Verification items for the finished model (mm, model axes). A direction names the side the tool comes from. Give positions to 0.01 mm unless a question says otherwise; leave off trailing zeros. Loops run counter-clockwise (first coordinate to the right, second up) from the corner with the lowest first, then second, coordinate; pieces in that order, holes last. Notation, with made-up numbers: (-25.5, 54.25) - (-19.5, 54.25) arc R17 cw to (-19.5, 74.25) - close; hole circle Ø6 at (89, -23.75). An arc over 180 degrees is marked (long way). One line per item, written item: value. Start each with the question number.
1. Scan lines: L1, parallel to Z at x = 0, y = 6.5; L2, parallel to X at y = 8, z = -195; L3, parallel to X at y = 7, z = 0. Record each from-to range of solid material in increasing order. Write a range as [from, to].
2. Access from +Z, -Z, +X, -X, +Y, -Y to the whole of each face (thin tool, end or side, straight path). Record for faces 5 (the flat face through (2, 3, 228)), 6 (the cylindrical face through (229, 2, 169)), 7 (the flat face through (120, 5, 231)).
3. Gauge pin test, flat ends, axial feed: pin 1 (13 mm diameter, centred on x = 0, z = -45, fed in from +Y); pin 2 (12 mm diameter, centred on x = -34, y = -54, fed in from +Z); pin 3 (5 mm diameter, centred on y = 7.5, z = -157, fed in from -X); pin 4 (11 mm diameter, centred on y = 5, z = -149, fed in from +X). Record the tip position at first contact, or that the pin passes through.
4. Sectioned sample at C-C (y = -34). Record the cut outline in (x, z), plus the area to 3 significant figures.
5. Mould release check, pull along X, two halves, no side actions. Record for faces 1 (the flat face through (228, 3, 163)), 2 (the flat face through (-120, 5, 231)), 3 (the cylindrical face through (-28, -49, -21)), 4 (the flat face through (-3, 5, 225)): pulls with the +X half, pulls with the -X half, needs draft (parallel to the pull), parting line crosses it, or undercut.
6. Sectioned sample at B-B (x = 12.5). Record the cut outline in (y, z).
7. Sectioned sample at A-A (z = 24). Record the cut outline in (x, y).
8. Sectioned sample at D-D (z = 75). Record the cut outline in (x, y).
from build123d import *

# Parameters (mm, degrees)
CROQUIS1_W              = 450
CROQUIS1_H              = 450
CROQUIS1_R              = 30
CROQUIS1_R_2            = 55
SALIENTE_EXTRUIR1_DEPTH = 10
CROQUIS7_R              = 4
CORTAR_EXTRUIR6_DEPTH   = 11
CROQUIS8_R              = 60
CROQUIS8_R_2            = 55
CORTAR_EXTRUIR7_DEPTH   = 5
CROQUIS9_R              = 55
CORTAR_EXTRUIR8_DEPTH   = 11
CROQUIS10_R             = 35
CROQUIS10_R_2           = 30
SALIENTE_EXTRUIR2_DEPTH = 100
CROQUIS11_R             = 2.5
SALIENTE_EXTRUIR3_DEPTH = 3
CROQUIS12_R             = 5
SALIENTE_EXTRUIR4_DEPTH = 3
CROQUIS14_R             = 2.5
SALIENTE_EXTRUIR5_DEPTH = 3
CROQUIS15_R             = 5
SALIENTE_EXTRUIR6_DEPTH = 3


with BuildPart() as part:
    # Croquis1 → Saliente-Extruir1 (new body)
    with BuildSketch(Plane(origin=(0, 0, 0), x_dir=(1, 0, 0), z_dir=(0, 1, 0))):
        Rectangle(CROQUIS1_W, CROQUIS1_H)
        Circle(CROQUIS1_R, mode=Mode.SUBTRACT)
        with Locations((0, 120)):
            Circle(CROQUIS1_R_2, mode=Mode.SUBTRACT)
    extrude(amount=SALIENTE_EXTRUIR1_DEPTH)

    # Croquis7 → Cortar-Extruir6 (cut, through all)
    with BuildSketch(Plane(origin=(0, 10, 0), x_dir=(1, 0, 0), z_dir=(0, 1, 0))):
        with Locations((-195, 195)):
            Circle(CROQUIS7_R)
        with Locations((195, 195)):
            Circle(CROQUIS7_R)
        with Locations((195, -195)):
            Circle(CROQUIS7_R)
        with Locations((-195, -195)):
            Circle(CROQUIS7_R)
        with Locations((-45, 0)):
            Circle(CROQUIS7_R)
        with Locations((0, 45)):
            Circle(CROQUIS7_R)
        with Locations((0, -45)):
            Circle(CROQUIS7_R)
        with Locations((45, 0)):
            Circle(CROQUIS7_R)
        with Locations((-187.5, 120)):
            Circle(CROQUIS7_R)
        with Locations((187.5, 120)):
            Circle(CROQUIS7_R)
    extrude(amount=-CORTAR_EXTRUIR6_DEPTH, mode=Mode.SUBTRACT)

    # Croquis8 → Cortar-Extruir7 (cut)
    with BuildSketch(Plane(origin=(0, 10, 0), x_dir=(1, 0, 0), z_dir=(0, 1, 0))):
        with Locations((0, 120)):
            Circle(CROQUIS8_R)
        with Locations((0, 120)):
            Circle(CROQUIS8_R_2, mode=Mode.SUBTRACT)
    extrude(amount=-CORTAR_EXTRUIR7_DEPTH, mode=Mode.SUBTRACT)

    # Croquis9 → Cortar-Extruir8 (cut, through all)
    with BuildSketch(Plane(origin=(0, 10, 0), x_dir=(1, 0, 0), z_dir=(0, 1, 0))):
        with Locations((0, 120)):
            Circle(CROQUIS9_R)
        Polygon((0, 120), (55, 120), (55, 225), (-55, 225), (-55, 120), align=None)
    extrude(amount=-CORTAR_EXTRUIR8_DEPTH, mode=Mode.SUBTRACT)

    # Croquis10 → Saliente-Extruir2 (add)
    with BuildSketch(Plane.XZ):
        Circle(CROQUIS10_R)
        Circle(CROQUIS10_R_2, mode=Mode.SUBTRACT)
    extrude(amount=SALIENTE_EXTRUIR2_DEPTH)

    # Croquis11 → Saliente-Extruir3 (add)
    with BuildSketch(Plane(origin=(225, 0, 0), x_dir=(0, 0, -1), z_dir=(1, 0, 0))):
        with Locations((-165, 5)):
            Circle(CROQUIS11_R)
        with Locations((-95, 5)):
            Circle(CROQUIS11_R)
    saliente_extruir3 = extrude(amount=SALIENTE_EXTRUIR3_DEPTH)

    # Croquis12 → Saliente-Extruir4 (add)
    with BuildSketch(Plane(origin=(228, 0, 0), x_dir=(0, 0, -1), z_dir=(1, 0, 0))):
        with Locations((-165, 5)):
            Circle(CROQUIS12_R)
        with Locations((-95, 5)):
            Circle(CROQUIS12_R)
    saliente_extruir4 = extrude(amount=SALIENTE_EXTRUIR4_DEPTH)

    # Simetría1: Saliente-Extruir3, Saliente-Extruir4 across plane
    add(saliente_extruir3.mirror(Plane(origin=(0, 0, 0), x_dir=(0, 0, 1), z_dir=(1, 0, 0))))
    add(saliente_extruir4.mirror(Plane(origin=(0, 0, 0), x_dir=(0, 0, 1), z_dir=(1, 0, 0))))

    # Croquis14 → Saliente-Extruir5 (add)
    with BuildSketch(Plane.XY.offset(225)):
        with Locations((-120, 5)):
            Circle(CROQUIS14_R)
        with Locations((0, 5)):
            Circle(CROQUIS14_R)
        with Locations((120, 5)):
            Circle(CROQUIS14_R)
    extrude(amount=SALIENTE_EXTRUIR5_DEPTH)

    # Croquis15 → Saliente-Extruir6 (add)
    with BuildSketch(Plane.XY.offset(228)):
        with Locations((-120, 5)):
            Circle(CROQUIS15_R)
        with Locations((0, 5)):
            Circle(CROQUIS15_R)
        with Locations((120, 5)):
            Circle(CROQUIS15_R)
    extrude(amount=SALIENTE_EXTRUIR6_DEPTH)


solid = part.part
Results are:
1. L1: z = [-60, -49], [-41, -30], [30, 41], [49, 231]
1. L2: x = [-225, -199], [-191, -55], [55, 191], [199, 225]
1. L3: x = [-225, -49], [-41, -30], [30, 41], [49, 225]
2. face 5: none
2. face 6: +X
2. face 7: +Z, +X, -X, +Y, -Y
3. pin 1: stops at y = 10
3. pin 2: stops at z = 21
3. pin 3: stops at x = -225
3. pin 4: stops at x = 225
4. outline: circle Ø70 at (0, 0); hole circle Ø60 at (0, 0)
4. area: 1,020 mm^2
5. face 1: undercut
5. face 2: needs draft
5. face 3: parting line crosses it
5. face 4: undercut
6. outline: (-100, -32.69) - (0, -32.69) - (0, -66.44) - (5, -66.44) - (5, -61.32) - (10, -61.32) - (10, -27.27) - (-100, -27.27) - close; (-100, 27.27) - (10, 27.27) - (10, 225) - (0, 225) - (0, 32.69) - (-100, 32.69) - close
7. outline: (-225, 0) - (-25.48, 0) - (-25.48, -100) - (-18, -100) - (-18, 10) - (-225, 10) - close; (18, -100) - (25.48, -100) - (25.48, 0) - (225, 0) - (225, 10) - (18, 10) - close
8. outline: (-225, 0) - (225, 0) - (225, 10) - (-225, 10) - close
